Autodesk Fusion 360 part; units mm, degrees
sketch "Sketch1" plane through (0, 0, 0) normal (1, 0, 0) x (0, 0, -1)
  line L0 (0, 0) -> (9, 0)
  line L1 (9, 0) -> (9, 5)
  line L2 (9, 5) -> (0, 5)
  line L3 (0, 5) -> (0, 0)
  line L4 (9, 0) -> (16.7782, -7.7782)
  line L5 (9, 0) -> (10, 0) construction
  line L6 (16.7782, -7.7782) -> (17.4853, -7.0711)
  line L7 (9, 0) -> (9.7071, 0.7071)
  line L8 (9.7071, 0.7071) -> (17.4853, -7.0711)
  line L9 (17.4853, -7.0711) -> (19.748, -4.8083)
  line L10 (16.7782, -7.7782) -> (18.1924, -9.1924)
  line L11 (19.748, -4.8083) -> (20.4551, -4.1012)
  line L12 (20.4551, -4.1012) -> (21.8693, -5.5154)
  line L13 (21.8693, -5.5154) -> (18.1924, -9.1924)
  line L14 (19.748, -4.8083) -> (11.9698, 2.9698)
  line L15 (11.9698, 2.9698) -> (9.7071, 0.7071)
  line L16 (20.4551, -4.1012) -> (11.3539, 5)
  line L17 (11.3539, 5) -> (9, 5)
  dimension "d1" = 9
  dimension "d2" = 5
  dimension "d3" = 45
  dimension "d4" = 11
  dimension "d5" = 1
  dimension "d6" = 1
  dimension "d7" = 3.2
  dimension "d8" = 2
  dimension "d9" = 1
  dimension "d10" = 2
extrude "Extrude1" add sketch "Sketch1" along normal blind 10 contours L0 L1 L2 L3 | L4 L6 L7 L8 | L1 L7 L11 L14 L15 L16 L17 | L6 L9 L10 L11 L12 L13
sketch "Sketch2" plane through (0, 0, 0) normal (0, -1, 0) x (1, 0, 0)
  line L0 (0, 0) -> (0, -9)
  line L1 (0, -9) -> (10, -9)
  line L2 (10, -9) -> (10, 0)
  line L3 (10, 0) -> (0, 0)
  circle A0 centre (5, -4.5) radius 2.5
  line L4 (0, -4.5) -> (5, -4.5)
  dimension "d13" = 5
extrude "Extrude2" cut sketch "Sketch2" against normal blind 5 contours A0
hole "Hole1" at (5, 0, -4.5) direction (0, 1, 0) diameter 8 depth 0.5 tip angle 118
fillet "Fillet1" radius 4 2 edges at (10, 2.5, 0) (0, 2.5, 0)
fillet "Fillet2" radius 5 1 edges at (5, 0, -9)
fillet "Fillet3" radius 8 1 edges at (5, 5, -11.3539)
fillet "Fillet4" radius 2 2 edges at (5, -9.1924, -18.1924) (5, -5.5154, -21.8693)
Design review of the part built by this model. Coordinates are the model's own, in mm. A direction names the side the tool comes from. Coordinates: 2 decimals unless noted, no trailing zeros. Loops run counter-clockwise (first coordinate to the right, second up) from the corner with the lowest first, then second, coordinate; pieces in that order, holes last. Notation, with made-up numbers: M -4,47 L 47,47 A23 cw 47,71 Z; hole C 7,-4 d2. An arc over 180 degrees is marked long. One line per question, with ' | ' between items.
(1) For pin 1 Ø4.5 at (x, z) = (5, -4.5) entering from -Y; pin 2 Ø2 at (x, y) = (9, 2) entering from +Z; pin 3 Ø4 at (x, z) = (2.5, -12) entering from -Y, all flat-tipped, find the tip position at first contact; note any pin that passes through.
Filled in:
pin 1: passes through | pin 2: stops at z = -0.54 | pin 3: stops at y = -5
(2) Draft analysis for pull direction Y (two halves, no side actions). For faces 1 (the face through (5.07, -5.54, -21.04)), 2 (the face through (7.385, 3.175, -3.749)), 3 (the face through (5, -4, -13)), 4 (the face through (4.93, -5.956, -18.601)), state which applies: released by +Y, released by -Y, zero draft, split by the parting line, or undercut.
Filled in:
face 1: split by the parting line | face 2: zero draft | face 3: released by -Y | face 4: undercut
(3) Machinability: for faces 5 (the face through (4.2, 0, -0.4)), 6 (the face through (8.905, 0.254, -3.633)), 7 (the face through (5, 2, -11)), which of the approach directions +Z, -Z, +X, -X, +Y, -Y give a long, thin tool a straight path to every point of the face, cutting with its end or side? Answer none if there is none.
Filled in:
face 5: +Z, +X, -X, -Y | face 6: -Y | face 7: +X, -X
(4) We need section B-B (y = -3.75). Give the boundary of the cut face in (x, z), and give its area (3 significant figures).
Filled in:
outline: M 0,-20.1 L 10,-20.1 L 10,-18.69 L 0,-18.69 Z; M 0,-14.16 L 10,-14.16 L 10,-12.75 L 0,-12.75 Z | area: 28.3 mm^2
(5) Wall thickness on probe 1 along X at (y, z) = (3.55, -4.5); probe 2 along Z at (x, y) = (5, 2.85); probe 3 along Z at (x, y) = (5, 2.8): over which ranges is each line inside the solid? List them lowest first.
Filled in:
probe 1: x = 0 to 2.5, 7.5 to 10 | probe 2: z = -13.5 to -12.09, -11.85 to -7, -2 to 0 | probe 3: z = -13.55 to -12.14, -11.8 to -7, -2 to 0
(6) We need section A-A (z = -4.5). Give the boundary of the cut face in (x, y), and give its area (3 significant figures).
Filled in:
outline: M 0,0 L 1,0 L 1,0.5 L 2.5,1.4 L 2.5,5 L 0,5 Z; M 7.5,1.4 L 9,0.5 L 9,0 L 10,0 L 10,5 L 7.5,5 Z | area: 22.1 mm^2
(7) We need section D-D (z = -13.25). Give the boundary of the cut face in (x, y), and give its area (3 significant figures).
Filled in:
outline: M 0,-4.25 L 10,-4.25 L 10,-2.84 L 0,-2.84 Z; M 0,1.69 L 10,1.69 L 10,3.07 L 0,3.07 Z | area: 28.0 mm^2
(8) We need section C-C (x = 3.5). Count the separate pieces of the cut face and the enclosed holes in it, and give its area (3 significant figures).
Filled in:
separate pieces: 2 | enclosed holes: 1 | area: 61.9 mm^2
